Autodesk Inventor part; units mm, degrees
ref_plane "YZ Plane" through (0, 0, 0) normal (1, 0, 0) x (0, 1, 0)
ref_plane "XZ Plane" through (0, 0, 0) normal (0, 1, 0) x (-1, 0, 0)
ref_plane "XY Plane" through (0, 0, 0) normal (0, 0, 1) x (1, 0, 0)
sketch "Sketch1" plane through (0, 0, 0) normal (1, 0, 0) x (0, 1, 0)
  line L0 (-58, -40) -> (-58, 50)
  line L1 (0, 0) -> (-57.3223, 54.5531) construction
  circle A0 centre (-23.5426, 22.4053) radius 7.5
  circle A1 centre (0, 0) radius 47 construction
  circle A2 centre (-43.4633, 41.3636) radius 7.5
  circle A3 centre (0, 0) radius 10
  line L2 (-11, -52) -> (14.1774, -52)
  line L3 (-58, 0) -> (-58, -40)
  line L4 (0, 0) -> (0, -52) construction
  line L5 (-58, -40) -> (-23, -52.739)
  circle A4 centre (0, 0) radius 50 construction
  arc A5 (22.2788, -50.2857) -> (0, 55) centre (0, 0) ccw
  line L6 (-43.4633, 41.3636) -> (-48.6337, 35.9307)
  arc A6 (-53, 55) -> (-58, 50) centre (-53, 50) ccw
  line L7 (-11, 54) -> (-11, 50)
  line L8 (-12, 49) -> (-22, 49)
  line L9 (-23, 50) -> (-23, 54)
  line L10 (-53, 55) -> (-24, 55)
  line L11 (-10, 55) -> (0, 55)
  arc A7 (-23, 54) -> (-24, 55) centre (-24, 54) ccw
  arc A8 (-10, 55) -> (-11, 54) centre (-10, 54) ccw
  arc A9 (-12, 49) -> (-11, 50) centre (-12, 50) ccw
  arc A10 (-23, 50) -> (-22, 49) centre (-22, 50) ccw
  arc A11 (14.1774, -52) -> (22.2788, -50.2857) centre (14.1774, -32) ccw
  line L12 (-23, -49.5) -> (-23, -52.739)
  line L13 (-11, -52) -> (-11, -49.5)
  line L14 (-11.5, -49) -> (-22.5, -49)
  arc A12 (-11, -49.5) -> (-11.5, -49) centre (-11.5, -49.5) ccw
  arc A13 (-22.5, -49) -> (-23, -49.5) centre (-22.5, -49.5) ccw
  point P0 (-28.9755, 27.5757)
  point P1 (-57.7919, 55)
  point P2 (-58, 55)
  point P3 (-25.2108, 39.6663)
  point P4 (17.9165, -52)
  point P5 (-23, 55)
  point P6 (-11, 52)
  dimension "d4" = 94
  dimension "d6" = 15
  dimension "d7" = 15
  dimension "d3" = 32.5
  dimension "d8" = 60
  dimension "d9" = 20
  dimension "d13" = 52
  dimension "d20" = 100
  dimension "d31" = 55
  dimension "d34" = 58
  dimension "d52" = 5
  dimension "d54" = 47
  dimension "d56" = 1
  dimension "d59" = 20
  dimension "d60" = 12
  dimension "d61" = 6
  dimension "d65" = 0.5
  dimension "d69" = 95
  dimension "d72" = 110
  dimension "d73" = 3
  dimension "d74" = 12
extrude "Extrusion3" add sketch "Sketch1" along normal blind 1.5
fillet "Fillet1" radius 5 1 edges at (0.75, -58, -40)
fillet "Fillet2" radius 1.5 2 edges at (0.75, -23, -52.739) (0.75, -11, -52)
properties part number "InnerFlange27130914"
The listing builds one solid part. Answer for the finished solid, in the listing's coordinates (mm). Coordinates: 2 decimals unless noted, no trailing zeros. Order: outer loops, then holes, each group sorted by start corner. A loop starts at its lowest first (then second) coordinate and runs counter-clockwise, first axis right, second up.
Q1. A cutting plane is placed at A-A, the plane z = 0. Write down the section's boundary in (x, y).
Q2. A cutting plane is placed at D-D, the plane z = -43.5. Write down the section's boundary in (x, y).
Q3. A cutting plane is placed at C-C, the plane x = 1.1. Write down the section's boundary in (y, z).
Q4. Given P1, Ø0.5, axis at x = 0.5, z = -50, coming from the +Y side; P2, Ø0.8, axis at x = 1, y = -15, coming from the +Z side, each flat-ended and moving along its own axis, determine where each tip first touches the part or whether it passes through.
Q5. A cutting plane is placed at B-B, the plane y = 4. Write down the section's boundary in (x, z).
Q6. For a pull along Y with two mould halves and no side action, classify faces 1 (the face through (0.74, 53.58, 12.41)), 2 (the face through (0.74, -31.035, 22.076)), 3 (the face through (1.5, -15, 2)) as pulls with the +Y half, pulls with the -Y half, needs draft (parallel to the pull), parting line crosses it, or undercut.
Q7. Consider line 1 (Z direction, x = 0.85, y = -15); line 2 (Z direction, x = 1, y = -39); line 3 (Y direction, x = 1.25, z = 4.5). Determine where each line is inside the solid, lowest interval first.
Answers follow:
1. outline: (0, -58) - (1.5, -58) - (1.5, -10) - (0, -10) - close; (0, 10) - (1.5, 10) - (1.5, 55) - (0, 55) - close
2. outline: (0, -48.38) - (1.5, -48.38) - (1.5, 33.66) - (0, 33.66) - close
3. outline: (-58, -36.5) arc R5 ccw to (-54.71, -41.2) - (-25.01, -52.01) arc R1.5 ccw to (-23, -50.6) - (-23, -49.5) arc R0.5 cw to (-22.5, -49) - (-11.5, -49) arc R0.5 cw to (-11, -49.5) - (-11, -50.5) arc R1.5 ccw to (-9.5, -52) - (14.18, -52) arc R20 ccw to (22.28, -50.29) arc R55 ccw to (0, 55) - (-10, 55) arc R1 ccw to (-11, 54) - (-11, 50) arc R1 cw to (-12, 49) - (-22, 49) arc R1 cw to (-23, 50) - (-23, 54) arc R1 ccw to (-24, 55) - (-53, 55) arc R5 ccw to (-58, 50) - close; hole circle Ø15 at (-43.46, 41.36); hole circle Ø15 at (-23.54, 22.41); hole circle Ø20 at (0, 0)
4. P1: stops at y = 23.45
4. P2: stops at z = 49
5. outline: (0, -52) - (1.5, -52) - (1.5, -9.17) - (0, -9.17) - close; (0, 9.17) - (1.5, 9.17) - (1.5, 54.85) - (0, 54.85) - close
6. face 1: pulls with the +Y half
6. face 2: undercut
6. face 3: needs draft
7. line 1: z = -49 to 49
7. line 2: z = -46.92 to 35.34, 47.39 to 55
7. line 3: y = -58 to -8.93, 8.93 to 54.82
